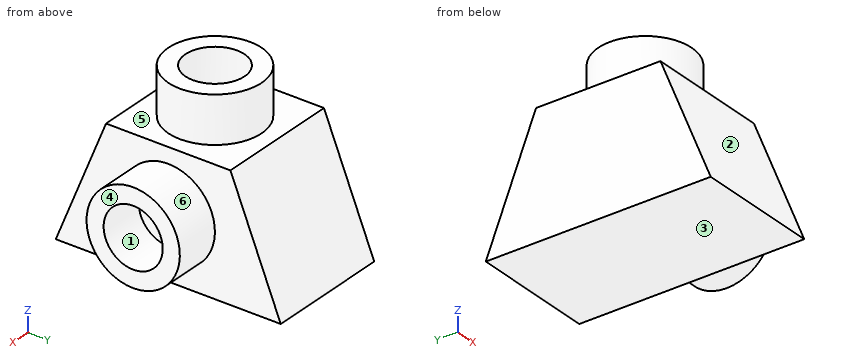
from build123d import *

# Parameters (mm, degrees)
CROQUIS1_R              = 30
CROQUIS1_R_2            = 19
SALIENTE_EXTRUIR1_DEPTH = 30
CROQUIS2_W              = 80
CROQUIS2_H              = 80
SALIENTE_EXTRUIR2_DEPTH = 80
CROQUIS3_R              = 30
CROQUIS3_R_2            = 19
SALIENTE_EXTRUIR3_DEPTH = 30
SALIENTE_EXTRUIR4_DEPTH = 80


with BuildPart() as part:
    # Croquis1 → Saliente-Extruir1 (new body)
    with BuildSketch(Plane.XY):
        Circle(CROQUIS1_R)
        Circle(CROQUIS1_R_2, mode=Mode.SUBTRACT)
    extrude(amount=SALIENTE_EXTRUIR1_DEPTH)

    # Croquis2 → Saliente-Extruir2 (add)
    with BuildSketch(Plane.XY):
        Rectangle(CROQUIS2_W, CROQUIS2_H)
    extrude(amount=-SALIENTE_EXTRUIR2_DEPTH)

    # Croquis3 → Saliente-Extruir3 (add)
    with BuildSketch(Plane(origin=(40, 0, 0), x_dir=(0, 0, -1), z_dir=(1, 0, 0))):
        with Locations((40, 0)):
            Circle(CROQUIS3_R)
        with Locations(Location((40, 0, 0), (0, 0, 90))):
            Circle(CROQUIS3_R_2, mode=Mode.SUBTRACT)
    extrude(amount=SALIENTE_EXTRUIR3_DEPTH)

    # Croquis4 → Saliente-Extruir4 (add)
    with BuildSketch(Plane(origin=(-40, 0, 0), x_dir=(0, 0, -1), z_dir=(1, 0, 0))):
        Polygon((80, 40), (80, 72.32), (0, 40), align=None)
        Polygon((0, -40), (80, -40), (80, -72.32), align=None)
    extrude(amount=SALIENTE_EXTRUIR4_DEPTH)


solid = part.part
Check sheet for the modelled part. Datum: model origin and axes. Units: mm. Face numbers are marked on the shaded views. A direction names the side the tool comes from. Give positions to 0.01 mm unless a question says otherwise; leave off trailing zeros. Loops run counter-clockwise (first coordinate to the right, second up) from the corner with the lowest first, then second, coordinate; pieces in that order, holes last. Notation, with made-up numbers: M 88,15.25 L 98,15.25 A25 ccw 98,28.25 Z; hole C 32,24 d10. An arc over 180 degrees is marked long. Answer as a JSON object with one key per item and string values. Group by question number.
Q1. Access from +Z, -Z, +X, -X, +Y, -Y to the whole of each face (thin tool, end or side, straight path). Record for the marked faces 4, 5 and 6.
Q2. Cross-section at C-C on z = 17. Record the cut outline in (x, y).
Q3. Cross-section at B-B on y = -24. Record the cut outline in (x, z).
Q4. Go/stop test with flat-tipped pins: P1, Ø3, axis at x = 27, z = -48, coming from the -Y side; P2, Ø1.5, axis at x = 18, z = -29, coming from the +Y side; P3, Ø5, axis at x = 31.5, y = -35.5, coming from the +Z side. Record where each tip stops, or that it passes through.
Q5. Release check for a two-part mould opening along Y. For the marked faces 1, 2 and 3 record: released by +Y, released by -Y, zero draft, split by the parting line, or undercut.
Q6. Material ranges on line 1 along X through (y, z) = (33.5, -70); line 2 along Y through (x, z) = (0, 19); line 3 along Z through (x, y) = (18.5, 62), recorded low to high. Write a range as [from, to].
Q7. Cross-section at D-D on x = 44. Record the cut outline in (y, z).
Q8. Cross-section at A-A on x = 0. Record the cut outline in (y, z).
Evaluation:
{
 "1": {"face 4": "+Z, -Z, +X, +Y, -Y", "face 5": "+Z", "face 6": "+X"},
 "2": {"outline": "C 0,0 d60; hole C 0,0 d38"},
 "3": {"outline": "M -40,-80 L 40,-80 L 40,-58 L 70,-58 L 70,-22 L 40,-22 L 40,0 L 18,0 L 18,30 L -18,30 L -18,0 L -40,0 Z"},
 "4": {"P1": "stops at y = -60", "P2": "stops at y = 52.02", "P3": "stops at z = 0"},
 "5": {"face 1": "undercut", "face 2": "released by -Y", "face 3": "zero draft"},
 "6": {"line 1": "x = [-40, 40]", "line 2": "y = [-30, -19], [19, 30]", "line 3": "z = [-80, -54.46]"},
 "7": {"outline": "C 0,-40 d60; hole C 0,-40 d38"},
 "8": {"outline": "M -72.32,-80 L 72.32,-80 L 40,0 L 30,0 L 30,30 L 19,30 L 19,0 L -19,0 L -19,30 L -30,30 L -30,0 L -40,0 Z"}
}
